Can you work these out from the drawing? Everything is in mm from the part's minimum corner. A direction names the side the tool comes from. Round coordinates to 2 decimals unless told otherwise and drop trailing zeros. Write each loop counter-clockwise with the first axis right and the second up, starting at its lowest first coordinate (ties: lowest second). Pieces come first, ordered by that corner, then holes. Notation, with made-up numbers: M 47.5,36.5 L 71.5,36.5 A16 cw 71.5,43.5 Z; hole C -40,15 d2. An arc over 180 degrees is marked long. Answer in a Markdown table with one row per item. Add a question column.
(1) I'm going to push flat-ended pins straight in: pin 1 (2 mm diameter, centred on y = 10.5, z = 5.5, fed in from -X); pin 2 (1 mm diameter, centred on y = 9, z = 3, fed in from -X) (1 decimal); pin 3 (4 mm diameter, centred on x = 2, y = 4.5, fed in from +Z) (3 decimals). Where does each tip first touch, or does it pass through?
(2) Suppose I cut it at D-D, the plane z = 4.75. Write out the boundary of the cut face in (x, y).
(3) For the marked faces 1 and 2, which set-ups out of +Z, -Z, +X, -X, +Y, -Y let a thin tool reach every point of the face, with its end or its side?
(4) Suppose I cut it at C-C, the plane z = 3.5. Write out the boundary of the cut face in (x, y), then the cut area to 3 significant figures.
(5) If I drill on probe 1 along Z at (x, y) = (9, 5.25) (1 decimal); probe 2 along Y at (x, z) = (4, 1.25); probe 3 along Z at (x, y) = (9.5, 12) (1 decimal), over which ranges is the centre line in solid material (lowest first)?
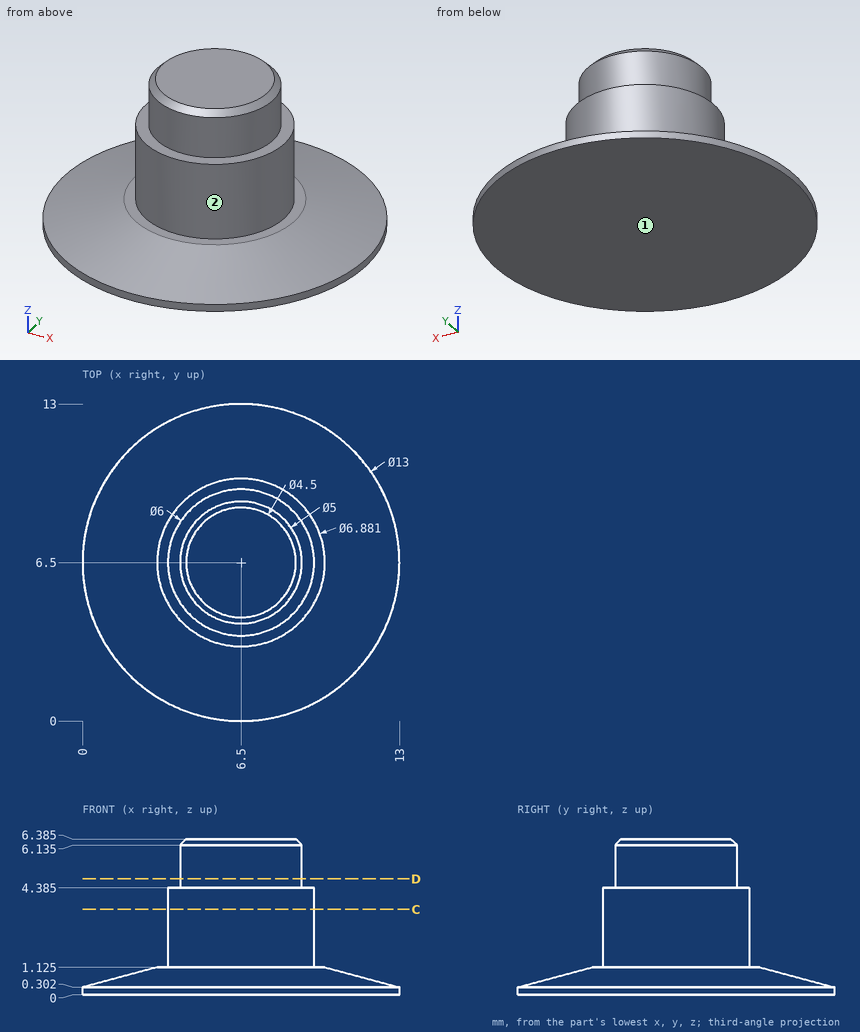
Calculated:
| question | item | result |
|---|---|---|
| 1 | pin 1 | through |
| 1 | pin 2 | x = 4.3 |
| 1 | pin 3 | z = 4.385 |
| 2 | outline | C 6.5,6.5 d5 |
| 3 | face 1 | -Z, +X, -X, +Y, -Y |
| 3 | face 2 | +Z |
| 4 | outline | C 6.5,6.5 d6 |
| 4 | area | 28.3 mm² |
| 5 | probe 1 | 0 to 4.4 |
| 5 | probe 2 | 4.84 to 8.16 |
| 5 | probe 3 | 0 to 0.4 |
